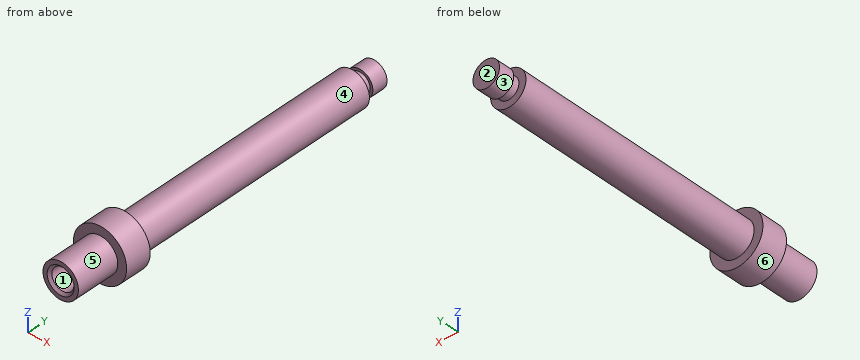
from build123d import *

# Parameters (mm, degrees)
TROU_TARAUD_M31_D           = 2.5
TROU_TARAUD_M31_DEPTH       = 8.5
TROU_TARAUD_M31_CSINK_D     = 3.05
TROU_TARAUD_M31_CSINK_ANGLE = 90
TROU_TARAUD_M31_TIP         = 0.751075774


with BuildPart() as part:
    # Esquisse1 → Révolution1 (revolve)
    with BuildSketch(Plane.XY):
        Polygon((0, 0), (-0.5, 0), (-0.5, -29), (-1.5, -29), (-1.5, -32), (-0.5, -32), (-0.5, -37), (1.5, -37), (1.5, 2.8), (0, 2.8), (0, 1), (0.3, 1), (0.3, 0), align=None)
    revolve(axis=Axis((1.5, -37, 0), (0, 1, 0)))

    # Trou taraudé M31
    with Locations(Plane(origin=(0, -37, 0), x_dir=(-1, 0, 0), z_dir=(0, -1, 0))):
        with Locations((-1.5, 0)):
            CounterSinkHole(TROU_TARAUD_M31_D / 2, TROU_TARAUD_M31_CSINK_D / 2, depth=TROU_TARAUD_M31_DEPTH, counter_sink_angle=TROU_TARAUD_M31_CSINK_ANGLE)
            with Locations((0, 0, -(TROU_TARAUD_M31_DEPTH + TROU_TARAUD_M31_TIP / 2))):  # 118° drill point
                Cone(0, TROU_TARAUD_M31_D / 2, TROU_TARAUD_M31_TIP, mode=Mode.SUBTRACT)


solid = part.part
Build history of the part. All positions in model axes, mm. Face numbers are marked on the shaded views. A direction names the side the tool comes from. Give positions to 0.01 mm unless a question says otherwise; leave off trailing zeros. Order: outer loops, then holes, each group sorted by start corner. A loop starts at its lowest first (then second) coordinate and runs counter-clockwise, first axis right, second up. Notation, with made-up numbers: M 55,3 L 69,3 A19 ccw 69,17 Z; hole C 33,48.5 d5. An arc over 180 degrees is marked long. Put each result on its own line as item: value.
Item 1: Cut at A-A on y = -29.5. Write the cut outline in (x, z).
Results are:
outline: C 1.5,0 d6; hole C 1.5,0 d2.5
Item 2: Drop flat-ended pins along their axis: pin 1 Ø0.9 at (x, z) = (1, 0.5) entering from -Y; pin 2 Ø1.5 at (x, z) = (-0.5, -1.5) entering from +Y; pin 3 Ø1 at (x, y) = (-0.5, -30.5) entering from +Z. Give the stop position or say it passes through.
Results are:
pin 1: y = -28.44
pin 2: y = 0
pin 3: z = 2.6
Item 3: Which spindle directions (+Z, -Z, +X, -X, +Y, -Y) get a long thin tool onto all of the face, cutting with end or side? Do the marked faces 4, 5 and 6. Say none if no direction does.
Results are:
face 4: +Y
face 5: -Y
face 6: +Y, -Y
Item 4: Cut at C-C on y = -20. Write the cut outline in (x, z), then the cut area to 3 significant figures.
Results are:
outline: C 1.5,0 d4
area: 12.6 mm2
Item 5: Pull direction Z, two halves, no side cores. Call the marked faces 1, 2 and 3: +Z half, -Z half, draft (parallel to the pull), parting line (faces both ways), or undercut.
Results are:
face 1: undercut
face 2: draft
face 3: parting line
Item 6: Cut at D-D on y = -34.5. Write the cut outline in (x, z).
Results are:
outline: C 1.5,0 d4; hole C 1.5,0 d2.5
Item 7: Wall check: probe 1 along Y at (x, z) = (3.45, 0.1); probe 2 along Z at (x, y) = (1.5, -31.5); probe 3 along Y at (x, z) = (4.2, 0.8). Give the ranges that are in metal, low to high.
Results are:
probe 1: -37 to 0
probe 2: -3 to -1.25, 1.25 to 3
probe 3: -32 to -29
Item 8: Cut at B-B on z = 2.65. Write the cut outline in (x, y), then the cut area to 3 significant figures.
Results are:
outline: M 0.09,-32 L 2.91,-32 L 2.91,-29 L 0.09,-29 Z
area: 8.44 mm2
